Geometry: final body of the model. Coordinates: model frame, mm. Face numbers are marked on the shaded views. A direction names the side the tool comes from. Round coordinates to 2 decimals unless told otherwise and drop trailing zeros. Loops run counter-clockwise (first coordinate to the right, second up) from the corner with the lowest first, then second, coordinate; pieces in that order, holes last. Notation, with made-up numbers: M 74.5,26 L 123.5,26 A24 ccw 123.5,47 Z; hole C -11.75,45 d6. An arc over 180 degrees is marked long. Return JSON: item names as keys, results as strings.
from build123d import *

# Parameters (mm, degrees)
F0_R     = 4
F1_DEPTH = 2
F2_W     = 3
F2_H     = 3
F3_DEPTH = 1


with BuildPart() as f1:
    # F0 (on Top) → F1 (new body)
    with BuildSketch(Plane.XY):
        Circle(F0_R)
    extrude(amount=-F1_DEPTH)

    # F2 (on face) → F3 (cut)
    with BuildSketch(Plane.XY):
        Rectangle(F2_W, F2_H)
    extrude(amount=-F3_DEPTH, mode=Mode.SUBTRACT)


solid = f1.part
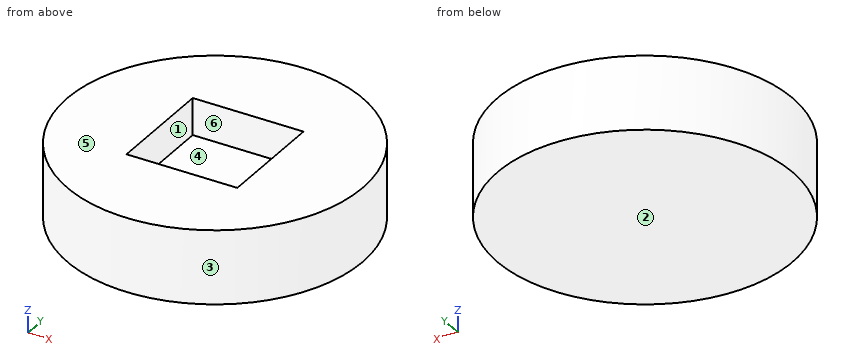
Q1. Material intervals for L1, parallel to X at y = -0.25, z = -0.95; L2, parallel to Z at x = 1, y = -1; L3, parallel to Y at x = 1.25, z = -0.35, sorted ascending.
Determined:
{"L1": "x = -3.99 to -1.5, 1.5 to 3.99", "L2": "z = -2 to -1", "L3": "y = -3.8 to -1.5, 1.5 to 3.8"}
Q2. Pin query (flat end, axial travel): pin 1 (1.1 mm diameter, centred on y = -0.5, z = -0.5, fed in from -X). Return the tip coordinate at first contact, or that it passes through.
Determined:
{"pin 1": "stops at x = -4"}
Q3. Section query A-A (x = 0). Output: boundary loops of the cut face in (y, z).
Determined:
{"outline": "M -4,-2 L 4,-2 L 4,0 L 1.5,0 L 1.5,-1 L -1.5,-1 L -1.5,0 L -4,0 Z"}
Q4. Section query C-C (z = -1.35). Output: boundary loops of the cut face in (x, y).
Determined:
{"outline": "C 0,0 d8"}
Q5. Section query D-D (x = -2.25). Output: boundary loops of the cut face in (y, z).
Determined:
{"outline": "M -3.31,-2 L 3.31,-2 L 3.31,0 L -3.31,0 Z"}
Q6. Pull-direction query (X, two-part tool) for the marked faces 3, 4, 5 and 6; classes: pulls with the +X half, pulls with the -X half, needs draft (parallel to the pull), parting line crosses it, or undercut.
Determined:
{"face 3": "parting line crosses it", "face 4": "undercut", "face 5": "needs draft", "face 6": "undercut"}
Q7. Reachability of the marked faces 1 and 2 from +Z, -Z, +X, -X, +Y, -Y: full face, straight path, thin tool, end or side. Return the list, or none.
Determined:
{"face 1": "+Z", "face 2": "-Z, +X, -X, +Y, -Y"}
